from build123d import *

# Parameters (mm, degrees)
SZKIC1_W                    = 10
SZKIC1_H                    = 8
SZKIC5_R                    = 6
DODANIE_WYCI_GNI_CIE1_DEPTH = 7.5


with BuildPart() as part:
    # Szkic1 → Obr_t1 (revolve)
    with BuildSketch(Plane.XY, mode=Mode.PRIVATE) as obr_t1_sk:
        with Locations((5, 4)):
            Rectangle(SZKIC1_W, SZKIC1_H)
    revolve(obr_t1_sk.sketch.rotate(Axis((10, 0, 0), (-1, 0, 0)), 270), axis=Axis((10, 0, 0), (-1, 0, 0)))

    # Szkic2 → Wyci_cie-obr_t1 (revolve, cut)
    with BuildSketch(Plane.XY, mode=Mode.PRIVATE) as wyci_cie_obr_t1_sk:
        with BuildLine():
            Line((0, 8), (0, 7.6))
            ThreePointArc((0, 7.6), (0.117157288, 7.882842712), (0.4, 8))
            Line((0.4, 8), (0, 8))
        make_face()
    revolve(wyci_cie_obr_t1_sk.sketch.rotate(Axis((10, 0, 0), (-1, 0, 0)), 270), axis=Axis((10, 0, 0), (-1, 0, 0)), mode=Mode.SUBTRACT)

    # Szkic3 → Obr_t2 (revolve)
    with BuildSketch(Plane.XY, mode=Mode.PRIVATE) as obr_t2_sk:
        Polygon((10, 0), (10, 5), (44.08, 5), (45, 4.08), (45, 0), align=None)
    revolve(obr_t2_sk.sketch.rotate(Axis((45, 0, 0), (-1, 0, 0)), 270), axis=Axis((45, 0, 0), (-1, 0, 0)))

    # Szkic4 → Wyci_cie-obr_t2 (revolve, cut)
    with BuildSketch(Plane.XY, mode=Mode.PRIVATE) as wyci_cie_obr_t2_sk:
        Polygon((0, 0), (0, 5.5), (5, 5.5), (8.175426481, 0), align=None)
    revolve(wyci_cie_obr_t2_sk.sketch.rotate(Axis((8.175426481, 0, 0), (-1, 0, 0)), 270), axis=Axis((8.175426481, 0, 0), (-1, 0, 0)), mode=Mode.SUBTRACT)

    # Szkic5 → Dodanie-wyci_gni_cie1 (add)
    with BuildSketch(Plane(origin=(0, 0, 0), x_dir=(0, 0, -1), z_dir=(1, 0, 0))):
        Circle(SZKIC5_R)
        Polygon((-4, 2.309401077), (-4, -2.309401077), (0, -4.618802154), (4, -2.309401077), (4, 2.309401077), (0, 4.618802154), align=None, mode=Mode.SUBTRACT)
    extrude(amount=DODANIE_WYCI_GNI_CIE1_DEPTH)


solid = part.part
Here's how the part is built. I have some questions about the finished solid (model axes, mm). A direction names the side the tool comes from. Round coordinates to 2 decimals unless told otherwise and drop trailing zeros. Order: outer loops, then holes, each group sorted by start corner. A loop starts at its lowest first (then second) coordinate and runs counter-clockwise, first axis right, second up. Notation, with made-up numbers: (-32.5, -33) -> (13.5, -33) arc R26 cw to (13.5, 0) -> close; hole circle Ø11 at (59.5, 78.5). An arc over 180 degrees is marked (long way). Return JSON: item names as keys, results as strings.
Q1. I need wall thicknesses on line 1 along Z through (x, y) = (3, 0.25); line 2 along Y through (x, z) = (13.5, -3); line 3 along X through (y, z) = (-6.25, 3.5). Which ranges of each line are inside material? Lowest first, please. Write a range as from..to.
Filled sheet:
{"line 1": "z = -8..-4, 4..8", "line 2": "y = -4..4", "line 3": "x = 0..10"}
Q2. For pin 1 Ø5 at (x, y) = (35, -4.5) entering from -Z; pin 2 Ø2 at (x, z) = (25, -2.5) entering from +Y; pin 3 Ø8 at (x, y) = (38.5, 5.5) entering from +Z; pin 4 Ø8 at (x, y) = (5.5, -2) entering from -Z, each with a flat end and sliding along its axis, tell me the tip position at first contact or that it passes through.
Filled sheet:
{"pin 1": "stops at z = -4.58", "pin 2": "stops at y = 4.77", "pin 3": "stops at z = 4.77", "pin 4": "stops at z = -8"}
Q3. If we mould it in two halves opening along Y, with no side actions, what happens to faces 4 (the flat face through (2.89, 3.48, 1.97)), 5 (the cylindrical face through (27.28, -4.88, -1.08)), 6 (the flat face through (45, 0, 0))? For each: released by +Y, released by -Y, zero draft, split by the parting line, or undercut.
Filled sheet:
{"face 4": "undercut", "face 5": "split by the parting line", "face 6": "zero draft"}
Q4. Which directions (+Z, -Z, +X, -X, +Y, -Y) give clear straight access to the entire face, cutting with the end or side of a thin tool? Please do faces 1 (the flat face through (0, -3.3, -3.3)), 2 (the flat face through (3, 0, 4)), 3 (the flat face through (10, -5.2, 0.1)).
Filled sheet:
{"face 1": "+Z, -Z, -X, +Y, -Y", "face 2": "-X", "face 3": "+X"}
Q5. If we section it at A-A on x = 3: List the corners of the cut face in (y, z) for me.
Filled sheet:
{"outline": "circle Ø16 at (0, 0); hole (-4.62, 0) -> (-2.31, -4) -> (2.31, -4) -> (4.62, 0) -> (2.31, 4) -> (-2.31, 4) -> close"}
Q6. If we section it at B-B on x = 12.5: List the corners of the cut face in (y, z) for me.
Filled sheet:
{"outline": "circle Ø10 at (0, 0)"}
